```python
from build123d import *

# Parameters (mm, degrees)
F1_DEPTH = 12.7
F3_DEPTH = 12.7
F5_DEPTH = 12.7
F7_R     = 6.35
F8_DEPTH = 63.5


with BuildPart() as f1:
    # F0 (on Front) → F1 (new body, symmetric)
    with BuildSketch(Plane.XZ):
        Polygon((31.5395204871, 76.1431381106), (-31.5395204871, 76.1431381106), (-76.1431381106, 31.5395204871), (-76.1431381106, -31.5395204871), (-31.5395204871, -76.1431381106), (31.5395204871, -76.1431381106), (76.1431381106, -31.5395204871), (76.1431381106, 31.5395204871), align=None)
    extrude(amount=F1_DEPTH, both=True)

    # F2 (on Top) → F3 (join, symmetric)
    with BuildSketch(Plane.XY):
        Polygon((-31.5866271988, -76.2568637729), (31.5866271988, -76.2568637729), (76.2568637729, -31.5866271988), (76.2568637729, 31.5866271988), (31.5866271988, 76.2568637729), (-31.5866271988, 76.2568637729), (-76.2568637729, 31.5866271988), (-76.2568637729, -31.5866271988), align=None)
    extrude(amount=F3_DEPTH, both=True)

    # F4 (on Right) → F5 (join, symmetric)
    with BuildSketch(Plane.YZ):
        Polygon((31.5395204871, 76.1431381106), (-31.5395204871, 76.1431381106), (-76.1431381106, 31.5395204871), (-76.1431381106, -31.5395204871), (-31.5395204871, -76.1431381106), (31.5395204871, -76.1431381106), (76.1431381106, -31.5395204871), (76.1431381106, 31.5395204871), align=None)
    extrude(amount=F5_DEPTH, both=True)

    # F7 (on 3pt) → F8 (cut, symmetric)
    with BuildSketch(Plane(origin=(0, 0, 0), x_dir=(0.7071067812, 0.7071067812, 0), z_dir=(0.7071067812, -0.7071067812, 0))):
        with Locations((0, 66.614896059)):
            Circle(F7_R)
    extrude(amount=F8_DEPTH, both=True, mode=Mode.SUBTRACT)


solid = f1.part
```
Model file for the job. Use its own axes, mm. A direction names the side the tool comes from. Give positions to 0.01 mm unless a question says otherwise; leave off trailing zeros. Loops run counter-clockwise (first coordinate to the right, second up) from the corner with the lowest first, then second, coordinate; pieces in that order, holes last. Notation, with made-up numbers: (31, 40) - (36, 40) arc R17 ccw to (36, 44) - close; hole circle Ø10 at (83, -2.75). An arc over 180 degrees is marked (long way). One line per item, written item: value. Start each with the question number.
1. Pin check, flat tips, straight feed: pin 1 (3 mm diameter, centred on x = -49, z = 40, fed in from +Y); pin 2 (12 mm diameter, centred on x = 52.5, y = -29, fed in from -Z); pin 3 (10 mm diameter, centred on y = 31.5, z = -22, fed in from -X). Stop position of each tip, or through.
2. Slice it at B-B (y = 27). List the corners of the cut face in (x, z).
3. Which spindle directions (+Z, -Z, +X, -X, +Y, -Y) get a long thin tool onto all of the face, cutting with end or side? Do faces 1 (the flat face through (12.7, -38, -37)), 2 (the flat face through (-38, -12.7, 38)), 3 (the flat face through (-38, 12.7, -37)), 4 (the flat face through (12.7, 37, -37)). Say none if no direction does.
4. Slice it at A-A (z = 6). List the corners of the cut face in (x, y).
5. Probe L1, parallel to X at y = -20.5, z = -27. List the from-to ranges inside material, lowest first. Write a range as from..to.
6. Pull direction Y, two halves, no side cores. Call faces 5 (the flat face through (-53.609, 54.234, 0.178)), 6 (the flat face through (-76.143, 0, -22)), 7 (the cylindrical face through (-4.24, -4.73, 66.89)): pulls with the +Y half, pulls with the -Y half, needs draft (parallel to the pull), parting line crosses it, or undercut.
Solution:
1. pin 1: stops at y = 12.7
1. pin 2: stops at z = -12.7
1. pin 3: stops at x = -12.7
2. outline: (-76.26, -12.7) - (-12.7, -12.7) - (-12.7, -76.14) - (12.7, -76.14) - (12.7, -12.7) - (76.26, -12.7) - (76.26, 12.7) - (12.7, 12.7) - (12.7, 76.14) - (-12.7, 76.14) - (-12.7, 12.7) - (-76.26, 12.7) - close
3. face 1: -Z, +X, -Y
3. face 2: +Z, -X, -Y
3. face 3: -Z, -X, +Y
3. face 4: -Z, +X, +Y
4. outline: (-76.26, -31.59) - (-31.59, -76.26) - (31.59, -76.26) - (76.26, -31.59) - (76.26, 31.59) - (31.59, 76.26) - (-31.59, 76.26) - (-76.26, 31.59) - close
5. L1: x = -12.7..12.7
6. face 5: pulls with the +Y half
6. face 6: needs draft
6. face 7: undercut
